from build123d import *

# Parameters (mm, degrees)
SCHIZZO1_W          = 11
SCHIZZO1_H          = 11
SCHIZZO1_W_2        = 9
SCHIZZO1_H_2        = 9
EXTRUDE_THIN1_DEPTH = 214.16
CHAMFER1_SIZE       = 0.5


with BuildPart() as part:
    # Schizzo1 → Extrude-Thin1 (new body)
    with BuildSketch(Plane.XY):
        with Locations((5.5, 5.5)):
            Rectangle(SCHIZZO1_W, SCHIZZO1_H)
        with Locations((5.5, 5.5)):
            Rectangle(SCHIZZO1_W_2, SCHIZZO1_H_2, mode=Mode.SUBTRACT)
    extrude(amount=EXTRUDE_THIN1_DEPTH)

    # Chamfer1
    chamfer1_edges = [part.edges().sort_by_distance(p)[0] for p in [
        (11, 11, 107.08),
        (0, 11, 107.08),
        (0, 0, 107.08),
        (11, 0, 107.08),
    ]]
    chamfer(chamfer1_edges, length=CHAMFER1_SIZE)


solid = part.part
Here's how the part is built. I have some questions about the finished solid (model axes, mm). A direction names the side the tool comes from. Coordinates: 2 decimals unless noted, no trailing zeros. Loops run counter-clockwise (first coordinate to the right, second up) from the corner with the lowest first, then second, coordinate; pieces in that order, holes last. Notation, with made-up numbers: (-8.75, 66.25) -> (25.25, 66.25) arc R15 ccw to (25.25, 74.25) -> close; hole circle Ø2 at (70.5, -17). An arc over 180 degrees is marked (long way). Use one line per item in the form item = value. Start each with the question number.
(1) If we section it at A-A (x = 5): Please give me the cut outline in (y, z), then the cut area to 3 significant figures.
(2) On a 3-axis mill with a long thin cutter (end or side, diameter ignored), from which of +Z, -Z, +X, -X, +Y, -Y can I reach the whole of each face in a straight line? I mean faces 4 (the face through (5, 1, 106)), 5 (the face through (0.5, 5.6, 0)). Say none if no direction works.
(3) We'd pull the mould along Y, two halves only. Please class faces 1 (the face through (0, 5, 106)), 2 (the face through (1, 5, 106)), 3 (the face through (5, 11, 106)): pulls with the +Y half, pulls with the -Y half, needs draft (parallel to the pull), parting line crosses it, or undercut.
(4) Please list where these lines run through material, in increasing order: line 1 along X through (y, z) = (1.75, 124.5); line 2 along X through (y, z) = (10.75, 195.5).
(5) If we section it at C-C (z = 169): Please give me the cut outline in (x, y), then the cut area to 3 significant figures.
Verdict:
q1.outline = (0, 0) -> (1, 0) -> (1, 214.16) -> (0, 214.16) -> close; (10, 0) -> (11, 0) -> (11, 214.16) -> (10, 214.16) -> close
q1.area = 428 mm²
q2.face_4 = +Z, -Z
q2.face_5 = -Z, +X, -X, +Y, -Y
q3.face_1 = needs draft
q3.face_2 = undercut
q3.face_3 = pulls with the +Y half
q4.line_1 = 0 to 1, 10 to 11
q4.line_2 = 0.25 to 10.75
q5.outline = (0, 0.5) -> (0.5, 0) -> (10.5, 0) -> (11, 0.5) -> (11, 10.5) -> (10.5, 11) -> (0.5, 11) -> (0, 10.5) -> close; hole (1, 1) -> (10, 1) -> (10, 10) -> (1, 10) -> close
q5.area = 39.5 mm²
